Source: CAD feature listing. Evaluate the final solid. Frame: model axes, mm. A direction names the side the tool comes from. Coordinates: 2 decimals unless noted, no trailing zeros. Loops run counter-clockwise (first coordinate to the right, second up) from the corner with the lowest first, then second, coordinate; pieces in that order, holes last. Notation, with made-up numbers: (45, 18.5) -> (50, 18.5) arc R31 cw to (50, 52.5) -> close; hole circle Ø2 at (75, 74). An arc over 180 degrees is marked (long way). Answer as CSV lines item,"result".
from build123d import *

# Parameters (mm, degrees)
F3_DEPTH = 20
F5_DEPTH = 7


with BuildPart() as f1:
    # F0 (on Front) → F1 (revolve)
    with BuildSketch(Plane.XZ):
        with BuildLine():
            Line((0, 0), (0, 8.53))
            ThreePointArc((0, 8.53), (-8.53, 0), (0, -8.53))
            Line((0, -8.53), (0, 0))
        make_face()
    revolve(axis=Axis((0, 0, 4.265), (0, 0, 1)))

    # F2 (on Front) → F3 (cut, symmetric)
    with BuildSketch(Plane.XZ):
        Polygon((-44.582818, 6.42), (0, 6.42), (47.697775, 6.42), (0, 28.326638), align=None)
    extrude(amount=F3_DEPTH, both=True, mode=Mode.SUBTRACT)

    # F4 (on face) → F5 (cut)
    with BuildSketch(Plane.XY.offset(6.42)):
        with BuildLine():
            ThreePointArc((1.151499, 2.386745), (-2.244323, -1.409083), (2.65, 0))
            ThreePointArc((2.65, 0), (2.244323, 1.409083), (1.151499, 2.386745))
        make_face()
    extrude(amount=-F5_DEPTH, mode=Mode.SUBTRACT)


solid = f1.part
(1) Cut plane B-B (z = 1.25). Return the cut outline in (x, y), then the cut area to 3 significant figures.
Computed values:
outline,"circle Ø16.88 at (0, 0); hole circle Ø5.3 at (0, 0)"
area,"202 mm^2"
(2) Material intervals for L1, parallel to X at y = 0, z = 4.25; L2, parallel to X at y = 0, z = 1.75; L3, parallel to Y at x = 2.25, z = 1.5, sorted ascending. Write a range as [from, to].
Computed values:
L1,"[-7.4, -2.65], [2.65, 7.4]"
L2,"[-8.35, -2.65], [2.65, 8.35]"
L3,"[-8.09, -1.4], [1.4, 8.09]"
(3) Pin query (flat end, axial travel): pin 1 Ø2.5 at (x, y) = (-0.5, -0.5) entering from +Z; pin 2 Ø6 at (x, z) = (5, -6) entering from +Y; pin 3 Ø6 at (y, z) = (-1.5, 4.5) entering from -X; pin 4 Ø3 at (x, y) = (1, 0) entering from -Z. Return the tip coordinate at first contact, or that it passes through.
Computed values:
pin 1,"z = -0.58"
pin 2,"y = 7.04"
pin 3,"x = -8.35"
pin 4,"z = -8.53"
(4) Access query for faces 1 (the flat face through (1, -3, 6.42)), 2 (the flat face through (0, 0, -0.58)). Directions: +Z, -Z, +X, -X, +Y, -Y. A direction counts if a zero-diameter tool reaches every point of the face in a straight line with its end or side. Return the directions, or none.
Computed values:
face 1,"+Z, +X, -X, +Y, -Y"
face 2,"+Z"
(5) Cut plane D-D (z = -2.5). Return the cut outline in (x, y).
Computed values:
outline,"circle Ø16.31 at (0, 0)"
(6) Cut plane C-C (y = 4.25). Return the cut outline in (x, z).
Computed values:
outline,"(-3.67, 6.42) arc R7.4 ccw (long way) to (3.67, 6.42) -> close"
(7) Cut plane A-A (x = 0). Return the cut outline in (y, z), then the cut area to 3 significant figures.
Computed values:
outline,"(-5.62, 6.42) arc R8.53 ccw (long way) to (5.62, 6.42) -> (2.65, 6.42) -> (2.65, -0.58) -> (-2.65, -0.58) -> (-2.65, 6.42) -> close"
area,"175 mm^2"
